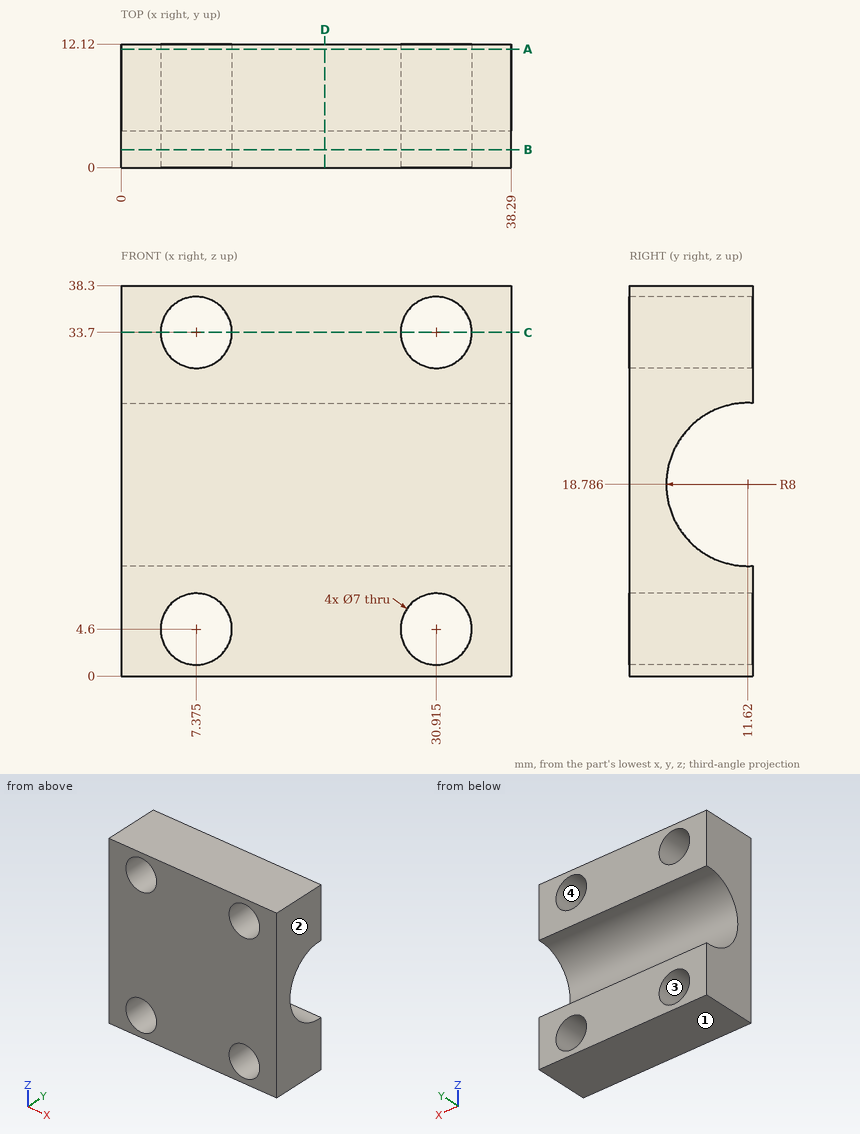
Input: dimensioned drawing with shaded views. Units: mm. Origin: part minimum x, y, z. Give positions to 0.01 mm unless a question says otherwise; leave off trailing zeros. Write each loop counter-clockwise with the first axis right and the second up, starting at its lowest first coordinate (ties: lowest second). Pieces come first, ordered by that corner, then holes.
1. Material intervals for line 1 along X through (y, z) = (4, 4.6) (3 decimals); line 2 along Z through (x, y) = (7.5, 3); line 3 along Z through (x, y) = (34, 9) (1 decimal), sorted ascending.
2. First-contact query: pin 1 (6 mm diameter, centred on x = 25.5, z = 10.5, fed in from -Y). Flat tip, straight axial feed; report the tip coordinate or a pass-through.
3. Pull-direction query (Z, two-part tool) for the marked faces 1, 2, 3 and 4; classes: +Z half, -Z half, draft (parallel to the pull), parting line (faces both ways), or undercut.
4. Section query D-D (x = 20). Return the cut outline in (y, z), then the cut area to 3 significant figures.
5. Section query C-C (z = 33.7). Return the cut outline in (x, y) (3 decimals), then the cut area to 3 significant figures.
6. Section query A-A (y = 11.62). Return the cut outline in (x, z) (1 decimal), then the cut area to 3 significant figures.
7. Section query B-B (y = 1.75). Return the cut outline in (x, z) (3 decimals).
Output values:
1. line 1: x = 0 to 3.875, 10.875 to 27.415, 34.415 to 38.29
1. line 2: z = 0 to 1.1, 8.1 to 30.2, 37.2 to 38.3
1. line 3: z = 0 to 2.9, 6.3 to 11.2, 26.3 to 32, 35.4 to 38.3
2. pin 1: stops at y = 0
3. face 1: -Z half
3. face 2: draft
3. face 3: undercut
3. face 4: undercut
4. outline: (0, 0) - (12.12, 0) - (12.12, 10.8) arc R8 cw (long way) to (12.12, 26.77) - (12.12, 38.3) - (0, 38.3) - close
4. area: 356 mm2
5. outline: (0, 0) - (3.875, 0) - (3.875, 12.12) - (0, 12.12) - close; (10.875, 0) - (27.415, 0) - (27.415, 12.12) - (10.875, 12.12) - close; (34.415, 0) - (38.29, 0) - (38.29, 12.12) - (34.415, 12.12) - close
5. area: 294 mm2
6. outline: (0, 0) - (38.3, 0) - (38.3, 10.8) - (0, 10.8) - close; (0, 26.8) - (38.3, 26.8) - (38.3, 38.3) - (0, 38.3) - close; hole circle Ø7 at (7.4, 4.6); hole circle Ø7 at (7.4, 33.7); hole circle Ø7 at (30.9, 4.6); hole circle Ø7 at (30.9, 33.7)
6. area: 700 mm2
7. outline: (0, 0) - (38.29, 0) - (38.29, 38.3) - (0, 38.3) - close; hole circle Ø7 at (7.375, 4.6); hole circle Ø7 at (7.375, 33.7); hole circle Ø7 at (30.915, 4.6); hole circle Ø7 at (30.915, 33.7)
